```python
from build123d import *

# Parameters (mm, degrees)
SKETCH1_W           = 101.6
SKETCH1_H           = 241.3
BOSS_EXTRUDE1_DEPTH = 3.175
SKETCH2_W           = 2.54
SKETCH2_H           = 5.08
SKETCH2_W_2         = 6.35
SKETCH2_H_2         = 2.54
CUT_EXTRUDE1_DEPTH  = 6.35
SKETCH3_W           = 6.35
SKETCH3_H           = 25.4
BOSS_EXTRUDE2_DEPTH = 3.175


with BuildPart() as part:
    # Sketch1 → Boss-Extrude1 (new body)
    with BuildSketch(Plane(origin=(0, 0, 0), x_dir=(1, 0, 0), z_dir=(0, 1, 0))):
        with Locations((50.8, 120.65)):
            Rectangle(SKETCH1_W, SKETCH1_H)
    extrude(amount=BOSS_EXTRUDE1_DEPTH)

    # Sketch2 → Cut-Extrude1 (cut)
    with BuildSketch(Plane(origin=(0, 3.175, 0), x_dir=(1, 0, 0), z_dir=(0, 1, 0))):
        with Locations((9.698538564, 20.940235373)):
            Rectangle(SKETCH2_W, SKETCH2_H)
        with Locations((9.698538564, 46.340235373)):
            Rectangle(SKETCH2_W, SKETCH2_H)
        with Locations((9.698538564, 71.740235373)):
            Rectangle(SKETCH2_W, SKETCH2_H)
        with Locations((9.698538564, 122.540235373)):
            Rectangle(SKETCH2_W, SKETCH2_H)
        with Locations((14.143538564, 173.828614979)):
            Rectangle(SKETCH2_W_2, SKETCH2_H_2)
        with Locations((14.143538564, 194.471385021)):
            Rectangle(SKETCH2_W_2, SKETCH2_H_2)
        with Locations((50.8, 193.04)):
            Rectangle(SKETCH2_W_2, SKETCH2_H_2)
        with Locations((50.8, 232.41)):
            Rectangle(SKETCH2_W_2, SKETCH2_H_2)
        Polygon((8.969375, 60.198), (0, 60.198), (0, 57.15), (8.969375, 57.15), (8.969375, 55.499), (11.350625, 55.499), (11.350625, 57.15), (17.78, 57.15), (17.78, 60.198), (11.350625, 60.198), (11.350625, 61.849), (8.969375, 61.849), align=None)
        Polygon((8.969375, 98.298), (0, 98.298), (0, 95.25), (8.969375, 95.25), (8.969375, 93.599), (11.350625, 93.599), (11.350625, 95.25), (17.78, 95.25), (17.78, 98.298), (11.350625, 98.298), (11.350625, 99.949), (8.969375, 99.949), align=None)
        Polygon((8.969375, 149.098), (0, 149.098), (0, 146.05), (8.969375, 146.05), (8.969375, 144.399), (11.350625, 144.399), (11.350625, 146.05), (17.78, 146.05), (17.78, 149.098), (11.350625, 149.098), (11.350625, 150.749), (8.969375, 150.749), align=None)
        Polygon((8.969375, 222.25), (0, 222.25), (0, 219.202), (8.969375, 219.202), (8.969375, 217.551), (11.350625, 217.551), (11.350625, 219.202), (17.78, 219.202), (17.78, 222.25), (11.350625, 222.25), (11.350625, 223.901), (8.969375, 223.901), align=None)
        with Locations((91.901461436, 20.940235373)):
            Rectangle(SKETCH2_W, SKETCH2_H)
        Polygon((90.249375, 61.849), (90.249375, 60.198), (83.82, 60.198), (83.82, 57.15), (90.249375, 57.15), (90.249375, 55.499), (92.630625, 55.499), (92.630625, 57.15), (101.6, 57.15), (101.6, 60.198), (92.630625, 60.198), (92.630625, 61.849), align=None)
        with Locations((91.901461436, 46.340235373)):
            Rectangle(SKETCH2_W, SKETCH2_H)
        with Locations((91.901461436, 71.740235373)):
            Rectangle(SKETCH2_W, SKETCH2_H)
        Polygon((90.249375, 93.599), (92.630625, 93.599), (92.630625, 95.25), (101.6, 95.25), (101.6, 98.298), (92.630625, 98.298), (92.630625, 99.949), (90.249375, 99.949), (90.249375, 98.298), (83.82, 98.298), (83.82, 95.25), (90.249375, 95.25), align=None)
        with Locations((91.901461436, 122.540235373)):
            Rectangle(SKETCH2_W, SKETCH2_H)
        Polygon((90.249375, 144.399), (92.630625, 144.399), (92.630625, 146.05), (101.6, 146.05), (101.6, 149.098), (92.630625, 149.098), (92.630625, 150.749), (90.249375, 150.749), (90.249375, 149.098), (83.82, 149.098), (83.82, 146.05), (90.249375, 146.05), align=None)
        Polygon((90.249375, 219.202), (90.249375, 217.551), (92.630625, 217.551), (92.630625, 219.202), (101.6, 219.202), (101.6, 222.25), (92.630625, 222.25), (92.630625, 223.901), (90.249375, 223.901), (90.249375, 222.25), (83.82, 222.25), (83.82, 219.202), align=None)
        with Locations((87.456461436, 194.471385021)):
            Rectangle(SKETCH2_W_2, SKETCH2_H_2)
        with Locations((87.456461436, 173.828614979)):
            Rectangle(SKETCH2_W_2, SKETCH2_H_2)
    extrude(amount=-CUT_EXTRUDE1_DEPTH, mode=Mode.SUBTRACT)

    # Sketch3 → Boss-Extrude2 (add)
    with BuildSketch(Plane(origin=(0, 3.175, 0), x_dir=(1, 0, 0), z_dir=(0, 1, 0))):
        with Locations((0, 187.452)):
            Rectangle(SKETCH3_W, SKETCH3_H)
        with Locations((0, 120.65)):
            Rectangle(SKETCH3_W, SKETCH3_H)
        with Locations((0, 76.2)):
            Rectangle(SKETCH3_W, SKETCH3_H)
        with Locations((0, 31.75)):
            Rectangle(SKETCH3_W, SKETCH3_H)
        with Locations((101.6, 31.75)):
            Rectangle(SKETCH3_W, SKETCH3_H)
        with Locations((101.6, 76.2)):
            Rectangle(SKETCH3_W, SKETCH3_H)
        with Locations((101.6, 120.65)):
            Rectangle(SKETCH3_W, SKETCH3_H)
        with Locations((101.6, 187.452)):
            Rectangle(SKETCH3_W, SKETCH3_H)
    extrude(amount=-BOSS_EXTRUDE2_DEPTH)


solid = part.part
```
The listing builds one solid part. Answer for the finished solid, in the listing's coordinates (mm). Coordinates: 2 decimals unless noted, no trailing zeros. Write each loop counter-clockwise with the first axis right and the second up, starting at its lowest first coordinate (ties: lowest second). Pieces come first, ordered by that corner, then holes. Notation, with made-up numbers: M 16,-1.5 L 20,-1.5 A12 cw 20,9.5 Z; hole C 0.5,62.5 d4. An arc over 180 degrees is marked long. Use a Markdown table: item, result. Add a question column.
1. Given P1, Ø0.8, axis at y = 1, z = -95, coming from the +X side; P2, Ø1.6, axis at x = 102.5, y = 1, coming from the -Z side; P3, Ø1.3, axis at y = 2.5, z = -99, coming from the -X side, each flat-ended and moving along its own axis, determine where each tip first touches the part or whether it passes through.
2. Section A-A (x = 96) is taken. Give the vertices of the cut face in (y, z) (3 decimals), plus the area to 3 significant figures.
3. Section C-C (z = -140) is taken. Give the vertices of the cut face in (x, y) (3 decimals).
4. Straight lines are drawn through the part: line 1 along Z through (x, y) = (98, 2.35); line 2 along X through (y, z) = (1.35, -71.5) (3 decimals); line 3 along X through (y, z) = (1.8, -48). For each, find the intervals that lie inside material, in ascending order. Write a range as [from, to].
5. Section B-B (y = 2.05) is taken. Count the separate pieces of the cut face and the enclosed holes in it, plus the area to 3 significant figures.
Data:
| question | item | result |
|---|---|---|
| 1 | P1 | stops at x = 101.6 |
| 1 | P2 | stops at z = -200.15 |
| 1 | P3 | stops at x = 0 |
| 2 | outline | M 0,-241.3 L 3.175,-241.3 L 3.175,-222.25 L 0,-222.25 Z; M 0,-219.202 L 3.175,-219.202 L 3.175,-149.098 L 0,-149.098 Z; M 0,-146.05 L 3.175,-146.05 L 3.175,-98.298 L 0,-98.298 Z; M 0,-95.25 L 3.175,-95.25 L 3.175,-60.198 L 0,-60.198 Z; M 0,-57.15 L 3.175,-57.15 L 3.175,0 L 0,0 Z |
| 2 | area | 727 mm2 |
| 3 | outline | M 0,0 L 101.6,0 L 101.6,3.175 L 0,3.175 Z |
| 4 | line 1 | z = [-241.3, -222.25], [-219.2, -149.1], [-146.05, -98.3], [-95.25, -60.2], [-57.15, 0] |
| 4 | line 2 | x = [-3.175, 8.429], [10.969, 90.631], [93.171, 104.775] |
| 4 | line 3 | x = [0, 8.43], [10.97, 90.63], [93.17, 101.6] |
| 5 | separate pieces | 1 |
| 5 | enclosed holes | 14 |
| 5 | area | 24,500 mm2 |
